from build123d import *

# Parameters (mm, degrees)
SKETCH3_W               = 50
SKETCH3_H               = 53.36450452
SKETCH3_W_2             = 45
SKETCH3_H_2             = 48.028054068
SKETCH6_W               = 50
SKETCH6_H               = 50
SKETCH6_W_2             = 45
SKETCH6_H_2             = 45
BOSS_EXTRUDE1_DEPTH     = 67.5
SKETCH8_W               = 50
SKETCH8_H               = 50
SKETCH8_W_2             = 45
SKETCH8_H_2             = 45
BOSS_EXTRUDE2_DEPTH     = 500
CUT_EXTRUDE1_DEPTH      = 728.345344386
CUT_EXTRUDE1_DEPTH_BACK = 728.345344386
SKETCH9_W               = 45
SKETCH9_H               = 45
SKETCH12_W              = 60
SKETCH12_H              = 115
SKETCH12_W_2            = 45
SKETCH12_H_2            = 48.028054068
BOSS_EXTRUDE6_DEPTH     = 5
SKETCH14_W              = 115
SKETCH14_H              = 55
BOSS_EXTRUDE7_DEPTH     = 5
SKETCH15_W              = 50
SKETCH15_H              = 50
SKETCH15_W_2            = 45
SKETCH15_H_2            = 45
BOSS_EXTRUDE8_DEPTH     = 1005
CUT_EXTRUDE3_DEPTH      = 1156.435523948
CUT_EXTRUDE3_DEPTH_BACK = 1156.435523948
SKETCH18_R              = 7
SKETCH19_R              = 7
BOSS_EXTRUDE9_DEPTH     = 2.5
CUT_EXTRUDE4_REACH      = 747.373
SKETCH20_R              = 5


with BuildPart() as part:
    # Sweep1: sweep along a path in Sketch1
    with BuildLine(Plane.XY) as sweep1_path:
        Line((0, 0), (0, 280))
        ThreePointArc((0, 280), (24.895923599, 340.104076401), (85, 365))
        Line((85, 365), (465, 365))
    # Sketch3 → Sweep1 (sweep)
    with BuildSketch(Plane(origin=(0, 0, 0), x_dir=(1, 0, 0), z_dir=(0, 1, 0))):
        Rectangle(SKETCH3_W, SKETCH3_H)
        Rectangle(SKETCH3_W_2, SKETCH3_H_2, mode=Mode.SUBTRACT)
    sweep(path=sweep1_path.line)

    # Sketch6 → Boss-Extrude1 (add)
    with BuildSketch(Plane.XY.offset(-25)):
        with Locations((130, 365)):
            Rectangle(SKETCH6_W, SKETCH6_H)
        with Locations((130, 365)):
            Rectangle(SKETCH6_W_2, SKETCH6_H_2, mode=Mode.SUBTRACT)
    boss_extrude1 = extrude(amount=-BOSS_EXTRUDE1_DEPTH)

    # Mirror1: Boss-Extrude1 across plane
    add(boss_extrude1.mirror(Plane.XY))

    # Sketch8 → Boss-Extrude2 (add)
    with BuildSketch(Plane(origin=(0, 0, 0), x_dir=(1, 0, 0), z_dir=(0, 1, 0))):
        with Locations((490, 0)):
            Rectangle(SKETCH8_W, SKETCH8_H)
        with Locations((490, 0)):
            Rectangle(SKETCH8_W_2, SKETCH8_H_2, mode=Mode.SUBTRACT)
    extrude(amount=BOSS_EXTRUDE2_DEPTH)

    # Sketch9 → Cut-Extrude1 (cut, two sides: drawn at the far end of the back side and taken through both)
    with BuildSketch(Plane.XY.offset(25).offset(-CUT_EXTRUDE1_DEPTH_BACK)):
        with Locations((130, 365)):
            Rectangle(SKETCH9_W, SKETCH9_H)
    extrude(amount=CUT_EXTRUDE1_DEPTH + CUT_EXTRUDE1_DEPTH_BACK, mode=Mode.SUBTRACT)

    # Sketch12 → Boss-Extrude6 (add)
    with BuildSketch(Plane(origin=(0, 0, 0), x_dir=(1, 0, 0), z_dir=(0, 1, 0))):
        Rectangle(SKETCH12_W, SKETCH12_H)
        Rectangle(SKETCH12_W_2, SKETCH12_H_2, mode=Mode.SUBTRACT)
    extrude(amount=-BOSS_EXTRUDE6_DEPTH)

    # Sketch14 → Boss-Extrude7 (add)
    with BuildSketch(Plane(origin=(-25, 0, 0), x_dir=(0, 0, -1), z_dir=(1, 0, 0))):
        with Locations((0, -27.5)):
            Rectangle(SKETCH14_W, SKETCH14_H)
    boss_extrude7 = extrude(amount=-BOSS_EXTRUDE7_DEPTH)

    # Mirror2: Boss-Extrude7 across plane
    add(boss_extrude7.mirror(Plane(origin=(0, 0, 0), x_dir=(0, 0, 1), z_dir=(1, 0, 0))))

    # Sketch15 → Boss-Extrude8 (add)
    with BuildSketch(Plane(origin=(30, 0, 0), x_dir=(0, 0, -1), z_dir=(1, 0, 0))):
        with Locations((0, -25)):
            Rectangle(SKETCH15_W, SKETCH15_H)
        with Locations((0, -25.38965636)):
            Rectangle(SKETCH15_W_2, SKETCH15_H_2, mode=Mode.SUBTRACT)
    extrude(amount=BOSS_EXTRUDE8_DEPTH)

    # Sketch18 → Cut-Extrude3 (cut, two sides: drawn at the far end of the back side and taken through both)
    with BuildSketch(Plane.XY.offset(25).offset(-CUT_EXTRUDE3_DEPTH_BACK)):
        with Locations(Location((640, -25, 0), (0, 0, 180))):
            Circle(SKETCH18_R)
        with Locations(Location((740, -25, 0), (0, 0, 180))):
            Circle(SKETCH18_R)
    extrude(amount=CUT_EXTRUDE3_DEPTH + CUT_EXTRUDE3_DEPTH_BACK, mode=Mode.SUBTRACT)

    # Sketch19 → Boss-Extrude9 (add, symmetric)
    # profile 1 of 2: a face of its own
    with BuildSketch(Plane(origin=(1035, 0, 0), x_dir=(0, 0, -1), z_dir=(1, 0, 0))):
        with BuildLine():
            Line((25, -50), (25, 0))
            Line((25, 0), (-25, 0))
            Line((-25, 0), (-26.68225226, 0))
            Line((-26.68225226, 0), (-39.279697572, 0))
            ThreePointArc((-39.279697572, 0), (-64.246269333, -24.966571761), (-39.279697572, -49.933143522))
            Line((-39.279697572, -49.933143522), (-25, -50))
            Line((-25, -50), (25, -50))
        make_face()
        with Locations((-45, -24.966571761)):
            Circle(SKETCH19_R, mode=Mode.SUBTRACT)
    # profile 2 of 2: a face of its own
    with BuildSketch(Plane(origin=(1035, 0, 0), x_dir=(0, 0, -1), z_dir=(1, 0, 0))):
        with BuildLine():
            Line((26.420207217, 0), (25, 0))
            Line((25, 0), (25, -50))
            Line((25, -50), (39.279697572, -49.933143522))
            ThreePointArc((39.279697572, -49.933143522), (64.246269333, -24.966571761), (39.279697572, 0))
            Line((39.279697572, 0), (26.68225226, 0))
            Line((26.68225226, 0), (26.420207217, 0))
        make_face()
        with Locations((45, -24.966571761)):
            Circle(SKETCH19_R, mode=Mode.SUBTRACT)
    extrude(amount=BOSS_EXTRUDE9_DEPTH, both=True)

    # Cut-Extrude4: up to this face of the body (flat: up to its plane)
    cut_extrude4_end = Plane(part.part.faces().sort_by_distance((465, 170, 0))[0])
    # Sketch20 → Cut-Extrude4 (cut, up to the picked face)
    with BuildSketch(Plane(origin=(515, 0, 0), x_dir=(0, 0, -1), z_dir=(1, 0, 0)), mode=Mode.PRIVATE) as cut_extrude4_sk1:
        with Locations((0, 150.748695463)):
            Circle(SKETCH20_R)
    cut_extrude4_tool1 = split(extrude(cut_extrude4_sk1.sketch, amount=-CUT_EXTRUDE4_REACH, mode=Mode.PRIVATE), bisect_by=cut_extrude4_end, keep=Keep.BOTH, mode=Mode.PRIVATE)
    add(cut_extrude4_tool1.solids().sort_by(Axis((515, 150.748695, 0), (-1, 0, 0)))[0], mode=Mode.SUBTRACT)


solid = part.part
Here's how the part is built. I have some questions about the finished solid (model axes, mm). A direction names the side the tool comes from. Coordinates: 2 decimals unless noted, no trailing zeros. Loops run counter-clockwise (first coordinate to the right, second up) from the corner with the lowest first, then second, coordinate; pieces in that order, holes last.
1. Imagine slicing it at C-C, the plane y = 428. Please give me the cut outline in (x, z), and give its area (3 significant figures).
2. For faces 1 (the flat face through (492, 40, -25)), 2 (the flat face through (4, -3, 57.5)), 3 (the flat face through (311, 365, 24.014)), which set-ups out of +Z, -Z, +X, -X, +Y, -Y let a thin tool reach every point of the face, with its end or its side?
3. Imagine slicing it at B-B, the plane x = 390. Please give me the cut outline in (y, z).
4. For P1, Ø13.5, axis at x = 497.5, z = -7, coming from the +Y side; P2, Ø6, axis at y = 18.5, z = -28.5, coming from the -X side; P3, Ø15, axis at x = 365.5, y = 360.5, coming from the +Z side, each with a flat end and sliding along its axis, tell me the tip position at first contact or that it passes through.
5. I need wall thicknesses on L1, parallel to Y at x = 248.5, z = 0.5; L2, parallel to X at y = 117, z = 3.5; L3, parallel to X at y = 359, z = -84.5. Which ranges of each line are inside material? Lowest first, please.
6. If we mould it in two halves opening along Z, with no side actions, what happens to faces 4 (the flat face through (107.5, 365, 58)), 5 (the flat face through (230, 342.5, 1)), 6 (the flat face through (128, 341, 92.5))? For each: pulls with the +Z half, pulls with the -Z half, needs draft (parallel to the pull), parting line crosses it, or undercut.
7. Imagine slicing it at A-A, the plane y = 256.5. Please give me the cut outline in (x, z), and give its area (3 significant figures).
8. Imagine slicing it at D-D, the plane x = 584. Please give me the cut outline in (y, z), and give its area (3 significant figures).
Taken from the geometry:
1. outline: (465, -25) - (515, -25) - (515, 25) - (465, 25) - close; hole (467.5, -22.5) - (512.5, -22.5) - (512.5, 22.5) - (467.5, 22.5) - close
1. area: 475 mm2
2. face 1: -Z, -Y
2. face 2: +Z, -X, +Y, -Y
2. face 3: none
3. outline: (-50, -25) - (0, -25) - (0, 25) - (-50, 25) - close; (340, -26.68) - (390, -26.68) - (390, 26.68) - (340, 26.68) - close; hole (-47.89, -22.5) - (-2.89, -22.5) - (-2.89, 22.5) - (-47.89, 22.5) - close; hole (342.5, -24.01) - (387.5, -24.01) - (387.5, 24.01) - (342.5, 24.01) - close
4. P1: stops at y = 0
4. P2: stops at x = -25
4. P3: stops at z = 26.68
5. L1: y = -50 to -47.89, -2.89 to 0, 340 to 342.5, 387.5 to 390
5. L2: x = -25 to -22.5, 22.5 to 25, 465 to 467.5, 512.5 to 515
5. L3: x = 105 to 107.5, 152.5 to 155
6. face 4: needs draft
6. face 5: undercut
6. face 6: pulls with the +Z half
7. outline: (-25, -26.68) - (25, -26.68) - (25, 26.68) - (-25, 26.68) - close; (465, -25) - (515, -25) - (515, 25) - (465, 25) - close; hole (-22.5, -24.01) - (22.5, -24.01) - (22.5, 24.01) - (-22.5, 24.01) - close; hole (467.5, -22.5) - (512.5, -22.5) - (512.5, 22.5) - (467.5, 22.5) - close
7. area: 982 mm2
8. outline: (-50, -25) - (0, -25) - (0, 25) - (-50, 25) - close; hole (-47.89, -22.5) - (-2.89, -22.5) - (-2.89, 22.5) - (-47.89, 22.5) - close
8. area: 475 mm2
